```python
from build123d import *

# Parameters (mm, degrees)
F0_W     = 10
F0_H     = 30
F1_DEPTH = 2
F2_R     = 2.202482
F2_R_2   = 0.557721
F3_DEPTH = 6
F4_R     = 3


with BuildPart() as f1:
    # F0 (on Top) → F1 (new body)
    with BuildSketch(Plane.XY):
        Rectangle(F0_W, F0_H)
    extrude(amount=F1_DEPTH)

    # F2 (on face) → F3 (join)
    with BuildSketch(Plane.XY.offset(2)):
        Circle(F2_R)
        Circle(F2_R_2, mode=Mode.SUBTRACT)
    extrude(amount=F3_DEPTH)

    # F4
    f4_edges = [f1.edges().sort_by_distance(p)[0] for p in [
        (5, 15, 1),
        (5, -15, 1),
        (-5, -15, 1),
        (-5, 15, 1),
    ]]
    fillet(f4_edges, radius=F4_R)


solid = f1.part
```
Build history of the part. All positions in model axes, mm. A direction names the side the tool comes from. Round coordinates to 2 decimals unless told otherwise and drop trailing zeros. Write each loop counter-clockwise with the first axis right and the second up, starting at its lowest first coordinate (ties: lowest second). Pieces come first, ordered by that corner, then holes. Notation, with made-up numbers: (78.5, 5.5) - (100.5, 5.5) arc R19 ccw to (100.5, 13.5) - close; hole circle Ø7 at (21.5, 77.25). An arc over 180 degrees is marked (long way). Write each question's results on one line, items separated by ' | '. Start each with the question number.
Item 1: Mould opens along Y. For faces 1 (the face through (-0.41, 0.38, 4.96)), 2 (the face through (5, 0, 1)), 3 (the face through (0, 15, 1)), 4 (the face through (4.1, -14.14, 1.01)) say: pulls with the +Y half, pulls with the -Y half, needs draft (parallel to the pull), parting line crosses it, or undercut.
Item 2: Which spindle directions (+Z, -Z, +X, -X, +Y, -Y) get a long thin tool onto all of the face, cutting with end or side? Do faces 5 (the face through (2.1, 0.66, 4.96)), 6 (the face through (-4.14, -14.1, 1.01)). Say none if no direction does.
Item 3: Saw through at B-B (y = 0). Write the cut outline in (x, z), and give its area (3 significant figures).
Item 4: Drop flat-ended pins along their axis: P1, Ø3, axis at y = -6, z = 4.5, coming from the -X side; P2, Ø1.5, axis at y = -1.5, z = 4, coming from the +X side; P3, Ø2, axis at x = 2, z = 6, coming from the -Y side; P4, Ø3, axis at x = 0, y = 8.5, coming from the +Z side. Give the stop position or say it passes through.
Item 5: Saw through at A-A (z = 6). Write the cut outline in (x, y).
Item 6: Wall check: L1, parallel to Y at x = 0, z = 4.6; L2, parallel to Z at x = 4.5, y = 8.25; L3, parallel to Y at x = -2.25, z = 1.5. Give the ranges that are in metal, low to high. Write a range as [from, to].
Item 7: Saw through at C-C (x = 0). Write the cut outline in (y, z).
Item 8: Saw through at D-D (y = 3.75). Write the cut outline in (x, z).
Results are:
1) face 1: undercut | face 2: needs draft | face 3: pulls with the +Y half | face 4: pulls with the -Y half
2) face 5: +Z | face 6: +Z, -Z, -X, -Y
3) outline: (-5, 0) - (5, 0) - (5, 2) - (2.2, 2) - (2.2, 8) - (0.56, 8) - (0.56, 2) - (-0.56, 2) - (-0.56, 8) - (-2.2, 8) - (-2.2, 2) - (-5, 2) - close | area: 39.7 mm²
4) P1: passes through | P2: stops at x = 2.07 | P3: stops at y = -1.96 | P4: stops at z = 2
5) outline: circle Ø4.4 at (0, 0); hole circle Ø1.12 at (0, 0)
6) L1: y = [-2.2, -0.56], [0.56, 2.2] | L2: z = [0, 2] | L3: y = [-14.99, 14.99]
7) outline: (-15, 0) - (15, 0) - (15, 2) - (2.2, 2) - (2.2, 8) - (0.56, 8) - (0.56, 2) - (-0.56, 2) - (-0.56, 8) - (-2.2, 8) - (-2.2, 2) - (-15, 2) - close
8) outline: (-5, 0) - (5, 0) - (5, 2) - (-5, 2) - close
